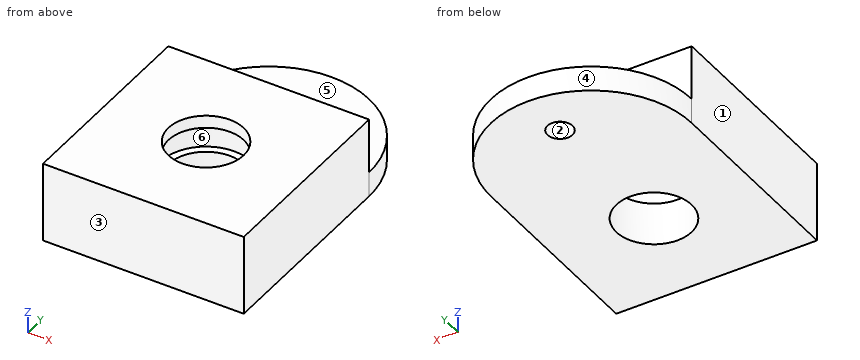
```python
from build123d import *

# Parameters (mm, degrees)
F1_DEPTH = 3.175
F2_W     = 25.4
F2_H     = 25.4
F3_DEPTH = 2.2098
F5_D     = 9.525
F6_W     = 25.4
F6_H     = 25.4
F6_R     = 5.715
F7_DEPTH = 3.175
F8_W     = 25.4
F8_H     = 25.4
F8_R     = 4.7625
F9_DEPTH = 1.6002
F11_D    = 3.175


with BuildPart() as f1:
    # F0 (on Top) → F1 (new body)
    with BuildSketch(Plane.XY):
        with BuildLine():
            Line((-12.7, -12.7), (12.7, -12.7))
            Line((12.7, -12.7), (12.7, 12.7))
            ThreePointArc((12.7, 12.7), (0, 25.4), (-12.7, 12.7))
            Line((-12.7, 12.7), (-12.7, -12.7))
        make_face()
    extrude(amount=F1_DEPTH)

    # F2 (on face) → F3 (join)
    with BuildSketch(Plane.XY.offset(3.175)):
        Rectangle(F2_W, F2_H)
    extrude(amount=F3_DEPTH)

    # F5 (through all)
    with Locations(Plane.XY.offset(5.3848)):
        with Locations((0, 0)):
            Hole(F5_D / 2)

    # F6 (on face) → F7 (join)
    with BuildSketch(Plane.XY.offset(5.3848)):
        Rectangle(F6_W, F6_H)
        Circle(F6_R, mode=Mode.SUBTRACT)
    extrude(amount=F7_DEPTH)

    # F8 (on face) → F9 (join)
    with BuildSketch(Plane.XY.offset(8.5598)):
        Rectangle(F8_W, F8_H)
        Circle(F8_R, mode=Mode.SUBTRACT)
    extrude(amount=F9_DEPTH)

    # F11 (through all)
    with Locations(Plane.XY.offset(3.175)):
        with Locations((0, 19.05)):
            Hole(F11_D / 2)


solid = f1.part
```
Can you work these out from the model? Positions are in its coordinate system, mm. Face numbers are marked on the shaded views. A direction names the side the tool comes from. Round coordinates to 2 decimals unless told otherwise and drop trailing zeros. Order: outer loops, then holes, each group sorted by start corner. A loop starts at its lowest first (then second) coordinate and runs counter-clockwise, first axis right, second up.
(1) If we section it at C-C (z = 2.75): Count the separate pieces of the cut face and the enclosed holes in it, plus the area to 3 significant figures.
Results are:
separate pieces: 1
enclosed holes: 2
area: 819 mm2
(2) We'd pull the mould along Y, two halves only. Please class the marked faces 1, 2 and 3: +Y half, -Y half, draft (parallel to the pull), parting line (faces both ways), or undercut.
Results are:
face 1: draft
face 2: undercut
face 3: -Y half
(3) If we section it at D-D (z = 5): Please give me the cut outline in (x, y) (1 decimal), plus the area to 3 significant figures.
Results are:
outline: (-12.7, -12.7) - (12.7, -12.7) - (12.7, 12.7) - (-12.7, 12.7) - close; hole circle Ø9.5 at (0, 0)
area: 574 mm2
(4) If we section it at B-B (x = 0): Please give me the cut outline in (y, z) (1 decimal), plus the area to 3 significant figures.
Results are:
outline: (-12.7, 0) - (-4.8, 0) - (-4.8, 5.4) - (-5.7, 5.4) - (-5.7, 8.6) - (-4.8, 8.6) - (-4.8, 10.2) - (-12.7, 10.2) - close; (4.8, 0) - (17.5, 0) - (17.5, 3.2) - (12.7, 3.2) - (12.7, 10.2) - (4.8, 10.2) - (4.8, 8.6) - (5.7, 8.6) - (5.7, 5.4) - (4.8, 5.4) - close; (20.6, 0) - (25.4, 0) - (25.4, 3.2) - (20.6, 3.2) - close
area: 185 mm2
(5) On a 3-axis mill with a long thin cutter (end or side, diameter ignored), from which of +Z, -Z, +X, -X, +Y, -Y can I reach the whole of each face in a straight line? I mean the marked faces 4, 5 and 6. Say none if no direction works.
Results are:
face 4: +Z, -Z, +Y
face 5: +Z, +X, -X, +Y
face 6: none
(6) I'm going to push flat-ended pins straight in: pin 1 (5 mm diameter, centred on x = 0, z = 8, fed in from +Y); pin 2 (4 mm diameter, centred on x = 5, y = 19, fed in from +Z) (3 decimals). Where does each tip first touch, or does it pass through?
Results are:
pin 1: stops at y = 12.7
pin 2: stops at z = 3.175
(7) If we section it at A-A (y = 0): Please give me the cut outline in (x, z) (1 decimal), plus the area to 3 significant figures.
Results are:
outline: (-12.7, 0) - (-4.8, 0) - (-4.8, 5.4) - (-5.7, 5.4) - (-5.7, 8.6) - (-4.8, 8.6) - (-4.8, 10.2) - (-12.7, 10.2) - close; (4.8, 0) - (12.7, 0) - (12.7, 10.2) - (4.8, 10.2) - (4.8, 8.6) - (5.7, 8.6) - (5.7, 5.4) - (4.8, 5.4) - close
area: 155 mm2
(8) If I drill on L1, parallel to Y at x = 0, z = 1.2; L2, parallel to Y at x = 0, z = 9.15; L3, parallel to Y at x = 10.75, z = 6.75, over which ranges is the centre line in solid material (lowest first)?
Results are:
L1: y = -12.7 to -4.76, 4.76 to 17.46, 20.64 to 25.4
L2: y = -12.7 to -4.76, 4.76 to 12.7
L3: y = -12.7 to 12.7
